The model under review builds one solid part; all positions refer to its coordinate system, in mm. A direction names the side the tool comes from. Coordinates: 2 decimals unless noted, no trailing zeros. Order: outer loops, then holes, each group sorted by start corner. A loop starts at its lowest first (then second) coordinate and runs counter-clockwise, first axis right, second up. Notation, with made-up numbers: (-8.5, 71) - (22.5, 71) arc R24 ccw to (22.5, 107) - close; hole circle Ø1 at (-27.75, 40). An arc over 180 degrees is marked (long way). Answer in a Markdown table with one row per item.
```python
from build123d import *

# Parameters (mm, degrees)
F0_R          = 0.5
F1_DEPTH      = 10
F0_R_2        = 1
F2_DEPTH      = 0.25
F3_R          = 0.15
F5_DEPTH      = 25
F5_DEPTH_BACK = 25
F7_DEPTH      = 25
F7_DEPTH_BACK = 25


with BuildPart() as f1:
    # F0 (on Top) → F1 (new body)
    with BuildSketch(Plane.XY):
        Circle(F0_R)
    extrude(amount=F1_DEPTH)

    # F0 (on Top) → F2 (join)
    with BuildSketch(Plane.XY):
        Circle(F0_R_2)
        Circle(F0_R, mode=Mode.SUBTRACT)
    extrude(amount=F2_DEPTH)

    # F3
    f3_edges = [f1.edges().sort_by_distance(p)[0] for p in [
        (-1, 0, 0),
    ]]
    fillet(f3_edges, radius=F3_R)

    # F4 (on Right) → F5 (cut, two sides)
    with BuildSketch(Plane.YZ) as f5_sk:
        Polygon((-0.642256, 9.187694), (0, 10.003787), (0.555127, 9.12749), (0.555127, 10.278048), (-0.642256, 10.278048), align=None)
    extrude(amount=F5_DEPTH, mode=Mode.SUBTRACT)
    extrude(f5_sk.sketch, amount=-F5_DEPTH_BACK, mode=Mode.SUBTRACT)

    # F6 (on Front) → F7 (cut, two sides)
    with BuildSketch(Plane.XZ) as f7_sk:
        Polygon((-0.578698, 9.359916), (0, 10.00354), (0.59532, 9.401632), (0.59532, 10.164445), (-0.578698, 10.164445), align=None)
    extrude(amount=F7_DEPTH, mode=Mode.SUBTRACT)
    extrude(f7_sk.sketch, amount=-F7_DEPTH_BACK, mode=Mode.SUBTRACT)


solid = f1.part
```
Item 1: To check wall thickness, follow line 1 (Z direction, x = 0.75, y = -0.3); line 2 (Z direction, x = -0.2, y = 0.25); line 3 (X direction, y = 0.05, z = 1.5). State the ranges of each line that lie inside material, in increasing order. Write a range as from..to.
Check values:
| item | result |
|---|---|
| line 1 | 0..0.25 |
| line 2 | 0..9.61 |
| line 3 | -0.5..0.5 |
Item 2: Tool access review of faces 1 (the face through (-0.108, -0.488, 4.864)), 2 (the face through (0, 0, 0)): name each direction out of +Z, -Z, +X, -X, +Y, -Y from which nothing blocks a thin tool from reaching the whole face with its end or side.
Check values:
| item | result |
|---|---|
| face 1 | +Z |
| face 2 | -Z, +X, -X, +Y, -Y |
Item 3: We need section A-A, the plane z = 5. Write out the cut boundary in (x, y), then the cut area to 3 significant figures.
Check values:
| item | result |
|---|---|
| outline | circle Ø1 at (0, 0) |
| area | 0.785 mm^2 |
